Geometry check sheet. Reference: the model listing, model coordinates, mm. A direction names the side the tool comes from. Give positions to 0.01 mm unless a question says otherwise; leave off trailing zeros. Write each loop counter-clockwise with the first axis right and the second up, starting at its lowest first coordinate (ties: lowest second). Pieces come first, ordered by that corner, then holes. Notation, with made-up numbers: (67, 63) - (105, 63) arc R21 cw to (105, 77) - close; hole circle Ø11 at (84.5, 6.5). An arc over 180 degrees is marked (long way). Use a Markdown table: item, result.
```python
from build123d import *

# Parameters (mm, degrees)
F0_W      = 70
F0_H      = 31
F1_DEPTH  = 1.5
F2_W      = 70
F2_H      = 3
F3_DEPTH  = 11
F4_W      = 70
F4_H      = 3
F5_DEPTH  = 11
F6_W      = 3.5
F6_H      = 25
F7_DEPTH  = 11
F8_W      = 3.5
F8_H      = 25
F9_DEPTH  = 11
F10_W     = 70
F10_H     = 17
F11_DEPTH = 15
F12_W     = 14
F12_H     = 5.5
F13_DEPTH = 70
F14_W     = 13
F14_H     = 5.5
F15_DEPTH = 70
F16_W     = 13
F16_H     = 5.5
F17_DEPTH = 70
F18_W     = 14
F18_H     = 5.5
F19_DEPTH = 70
F21_R     = 3.5
F22_DEPTH = 3.5
F23_R     = 3.5
F24_DEPTH = 3.5
F25_R     = 10
F26_DEPTH = 3
F27_R     = 10
F28_DEPTH = 3.5
F29_R     = 2.5
F30_DEPTH = 4
F31_R     = 2.5
F32_DEPTH = 4
F33_R     = 6.5
F34_DEPTH = 5.5


# Not quite as in the source:
# - a pattern or mirror of a feature is missing from the dataset's text; its kind, count and spacing are read off the source's solid


with BuildPart() as f1:
    # F0 (on Front) → F1 (new body, symmetric)
    with BuildSketch(Plane.XZ):
        Rectangle(F0_W, F0_H)
    extrude(amount=F1_DEPTH, both=True)

    # F2 (on face) → F3 (join)
    with BuildSketch(Plane.XZ.offset(1.5)):
        with Locations((0, -14)):
            Rectangle(F2_W, F2_H)
    extrude(amount=F3_DEPTH)

    # F4 (on face) → F5 (join)
    with BuildSketch(Plane.XZ.offset(1.5)):
        with Locations((0, 14)):
            Rectangle(F4_W, F4_H)
    extrude(amount=F5_DEPTH)

    # F6 (on face) → F7 (join)
    with BuildSketch(Plane.XZ.offset(1.5)):
        with Locations((33.25, 0)):
            Rectangle(F6_W, F6_H)
    extrude(amount=F7_DEPTH)

    # F8 (on face) → F9 (join)
    with BuildSketch(Plane.XZ.offset(1.5)):
        with Locations((-33.25, 0)):
            Rectangle(F8_W, F8_H)
    extrude(amount=F9_DEPTH)

    # F10 (on face) → F11 (join)
    with BuildSketch(Plane(origin=(0, 1.5, 0), x_dir=(-1, 0, 0), z_dir=(0, 1, 0))):
        Rectangle(F10_W, F10_H)
    extrude(amount=F11_DEPTH)

    # F12 (on face) → F13 (cut)
    with BuildSketch(Plane(origin=(0, 0, -15.5), x_dir=(1, 0, 0), z_dir=(0, 0, -1))):
        with Locations((24.5, 5.25)):
            Rectangle(F12_W, F12_H)
    extrude(amount=-F13_DEPTH, mode=Mode.SUBTRACT)

    # F14 (on face) → F15 (cut)
    with BuildSketch(Plane(origin=(0, 0, -15.5), x_dir=(1, 0, 0), z_dir=(0, 0, -1))):
        with Locations((8, 5.25)):
            Rectangle(F14_W, F14_H)
    extrude(amount=-F15_DEPTH, mode=Mode.SUBTRACT)

    # F16 (on face) → F17 (cut)
    with BuildSketch(Plane(origin=(0, 0, -15.5), x_dir=(1, 0, 0), z_dir=(0, 0, -1))):
        with Locations((-8, 5.25)):
            Rectangle(F16_W, F16_H)
    extrude(amount=-F17_DEPTH, mode=Mode.SUBTRACT)

    # F18 (on face) → F19 (cut)
    with BuildSketch(Plane(origin=(0, 0, -15.5), x_dir=(1, 0, 0), z_dir=(0, 0, -1))):
        with Locations((-24.5, 5.25)):
            Rectangle(F18_W, F18_H)
    extrude(amount=-F19_DEPTH, mode=Mode.SUBTRACT)

    # F21 (on face) → F22 (join)
    with BuildSketch(Plane.XY.offset(8.5)):
        with Locations((21.5, 13)):
            Circle(F21_R)
    f22 = extrude(amount=F22_DEPTH)

    # F22_copies: F22 across plane
    add(f22.mirror(Plane(origin=(0, 0, 0), x_dir=(-1, 0, 0), z_dir=(0, 0, -1))))

    # F23 (on face) → F24 (join)
    with BuildSketch(Plane.XY.offset(8.5)):
        with Locations((-22.1062030418, 13)):
            Circle(F23_R)
    f24 = extrude(amount=F24_DEPTH)

    # F24_copies: F24 across plane
    add(f24.mirror(Plane(origin=(0, 0, 0), x_dir=(-1, 0, 0), z_dir=(0, 0, -1))))

    # F25 (on face) → F26 (join)
    with BuildSketch(Plane.XY.offset(12)):
        with Locations((21.5, 13)):
            Circle(F25_R)
    f26 = extrude(amount=F26_DEPTH)

    # F26_copies: F26 across plane
    add(f26.mirror(Plane(origin=(0, 0, 0), x_dir=(-1, 0, 0), z_dir=(0, 0, -1))))

    # F27 (on face) → F28 (join)
    with BuildSketch(Plane.XY.offset(12)):
        with Locations((-22.1062030418, 13)):
            Circle(F27_R)
    f28 = extrude(amount=F28_DEPTH)

    # F28_copies: F28 across plane
    add(f28.mirror(Plane(origin=(0, 0, 0), x_dir=(-1, 0, 0), z_dir=(0, 0, -1))))

    # F29 (on face) → F30 (join)
    with BuildSketch(Plane.XY.offset(15.5)):
        with Locations((-22.1062030418, 13)):
            Circle(F29_R)
    f30 = extrude(amount=F30_DEPTH)

    # F30_copies: F30 across plane
    add(f30.mirror(Plane(origin=(0, 0, 0), x_dir=(-1, 0, 0), z_dir=(0, 0, -1))))

    # F31 (on face) → F32 (join)
    with BuildSketch(Plane.XY.offset(15)):
        with Locations((21.5, 13)):
            Circle(F31_R)
    f32 = extrude(amount=F32_DEPTH)

    # F32_copies: F32 across plane
    add(f32.mirror(Plane(origin=(0, 0, 0), x_dir=(-1, 0, 0), z_dir=(0, 0, -1))))

    # F33 (on face) → F34 (join)
    with BuildSketch(Plane(origin=(-35, 0, 0), x_dir=(0, -1, 0), z_dir=(-1, 0, 0))):
        with Locations((-9, 0)):
            Circle(F33_R)
    f34 = extrude(amount=F34_DEPTH)

    # F34_copies: F34 across plane
    add(f34.mirror(Plane(origin=(0, 0, 0), x_dir=(0, 0, 1), z_dir=(1, 0, 0))))

    # F35 (on face) → F36 (revolve)
    with BuildSketch(Plane(origin=(-40.5, 0, 0), x_dir=(0, -1, 0), z_dir=(-1, 0, 0))):
        with BuildLine():
            Line((-15.5, 0), (-9, 0))
            Line((-9, 0), (-2.5, 0))
            ThreePointArc((-2.5, 0), (-9, 6.5), (-15.5, 0))
        make_face()
    f36 = revolve(axis=Axis((-40.5, 9, 0), (0, 1, 0)))

    # F36_copies: F36 across plane
    add(f36.mirror(Plane(origin=(0, 0, 0), x_dir=(0, 0, 1), z_dir=(1, 0, 0))))


solid = f1.part
```
1) Section check C-C on x = -28. Record the boundary of the cut face in (y, z), then the cut area to 3 significant figures.
Working result:
| item | result |
|---|---|
| outline | (-12.5, -15.5) - (-8, -15.5) - (-8, -12.5) - (-12.5, -12.5) - close; (-12.5, 12.5) - (-8, 12.5) - (-8, 15.5) - (-12.5, 15.5) - close; (-2.5, -15.5) - (1.5, -15.5) - (1.5, -8.5) - (16.5, -8.5) - (16.5, 8.5) - (1.5, 8.5) - (1.5, 15.5) - (-2.5, 15.5) - (-2.5, 12.5) - (-1.5, 12.5) - (-1.5, -12.5) - (-2.5, -12.5) - close; (4.92, -15.5) - (21.08, -15.5) - (21.08, -12) - (4.92, -12) - close; (4.92, 12) - (21.08, 12) - (21.08, 15.5) - (4.92, 15.5) - close |
| area | 494 mm² |
2) Set-up check for faces 1 (the flat face through (-20, 11, -15.5)), 2 (the flat face through (-20, 11, 15.5)), 3 (the flat face through (21, 13, 19)), 4 (the flat face through (21, 9, 12)), 5 (the flat face through (-25, -8, 14)): record each of +Z, -Z, +X, -X, +Y, -Y from which the full face is reachable in a straight line by a thin tool's end or side.
Working result:
| item | result |
|---|---|
| face 1 | -Z |
| face 2 | +Z |
| face 3 | +Z, +X, +Y, -Y |
| face 4 | none |
| face 5 | +Z, -Z |
3) Mould release check, pull along Y, two halves, no side actions. Record for faces 6 (the flat face through (0, -5, 15.5)), 7 (the flat face through (-3, -12.5, -13)), 8 (the flat face through (14.5, -5, -14)): pulls with the +Y half, pulls with the -Y half, needs draft (parallel to the pull), parting line crosses it, or undercut.
Working result:
| item | result |
|---|---|
| face 6 | needs draft |
| face 7 | pulls with the -Y half |
| face 8 | undercut |
4) Section check A-A on x = 7. Record the boundary of the cut face in (y, z).
Working result:
| item | result |
|---|---|
| outline | (-12.5, -15.5) - (-8, -15.5) - (-8, -12.5) - (-12.5, -12.5) - close; (-12.5, 12.5) - (-8, 12.5) - (-8, 15.5) - (-12.5, 15.5) - close; (-2.5, -15.5) - (1.5, -15.5) - (1.5, -8.5) - (16.5, -8.5) - (16.5, 8.5) - (1.5, 8.5) - (1.5, 15.5) - (-2.5, 15.5) - (-2.5, 12.5) - (-1.5, 12.5) - (-1.5, -12.5) - (-2.5, -12.5) - close |
5) Section check B-B on z = 0. Record the boundary of the cut face in (x, y), then the cut area to 3 significant figures.
Working result:
| item | result |
|---|---|
| outline | (-40.5, 2.5) - (-35, 2.5) - (-35, -12.5) - (-31.5, -12.5) - (-31.5, -1.5) - (31.5, -1.5) - (31.5, -12.5) - (35, -12.5) - (35, 2.5) - (40.5, 2.5) arc R6.5 ccw to (40.5, 15.5) - (35, 15.5) - (35, 16.5) - (-35, 16.5) - (-35, 15.5) - (-40.5, 15.5) arc R6.5 ccw to start |
| area | 1,610 mm² |
6) Depth check by flat-ended pin: P1, Ø1.5, axis at y = -3.5, z = 14, coming from the +X side; P2, Ø2.5, axis at y = -6.5, z = -14, coming from the -X side; P3, Ø4, axis at x = -13, y = 4.5, coming from the +Z side. Enter the tip coordinate at first touch or a pass-through.
Working result:
| item | result |
|---|---|
| P1 | stops at x = 35 |
| P2 | stops at x = -35 |
| P3 | stops at z = 8.5 |
7) Section check D-D on y = 8. Record the boundary of the cut face in (x, z), then the cut area to 3 significant figures.
Working result:
| item | result |
|---|---|
| outline | (-40.5, -6.42) - (-35, -6.42) - (-35, -8.5) - (35, -8.5) - (35, -6.42) - (40.5, -6.42) arc R6.42 ccw to (40.5, 6.42) - (35, 6.42) - (35, 8.5) - (-35, 8.5) - (-35, 6.42) - (-40.5, 6.42) arc R6.42 ccw to start; (-30.77, -15.5) - (-13.45, -15.5) - (-13.45, -12) - (-30.77, -12) - close; (-30.77, 12) - (-13.45, 12) - (-13.45, 15.5) - (-30.77, 15.5) - close; (12.84, -15) - (30.16, -15) - (30.16, -12) - (12.84, -12) - close; (12.84, 12) - (30.16, 12) - (30.16, 15) - (12.84, 15) - close |
| area | 1,690 mm² |
8) Material ranges on L1, parallel to Y at x = 21, z = 14.5; L2, parallel to Y at x = -9, z = 15; L3, parallel to Z at x = -21, y = -2, recorded low to high. Write a range as from..to.
Working result:
| item | result |
|---|---|
| L1 | y = -12.5..-8, -2.5..1.5, 3.01..22.99 |
| L2 | y = -12.5..-8, -2.5..1.5 |
| L3 | z = -15.5..-12.5, 12.5..15.5 |
